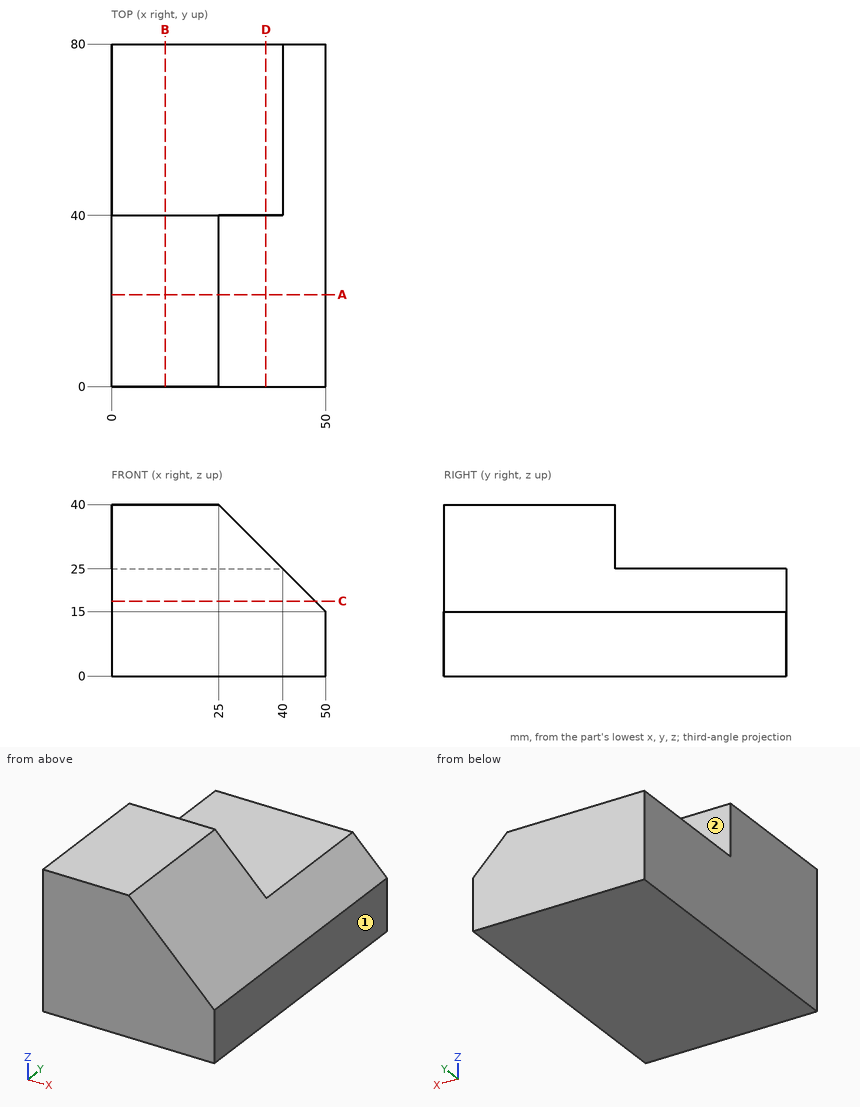
Design review of the part shown in the three views and the two pictorial views. Dimensions are in mm from the part's minimum x, y and z. A direction names the side the tool comes from. Give positions to 0.01 mm unless a question says otherwise; leave off trailing zeros. Write each loop counter-clockwise with the first axis right and the second up, starting at its lowest first coordinate (ties: lowest second). Pieces come first, ordered by that corner, then holes. Notation, with made-up numbers: M -31.75,-8.75 L 9.25,-8.75 A17 cw 9.25,4.25 Z; hole C -21,23 d3. An arc over 180 degrees is marked long. One line per question, with ' | ' between items. Start each with the question number.
Item 1: For the marked faces 1 and 2, list the 3-axis set-ups (+Z, -Z, +X, -X, +Y, -Y) from which the entire face can be reached by the end or side of a thin tool; tool diameter is ignored.
Item 2: For pin 1 (2 mm diameter, centred on y = 58.5, z = 24.5, fed in from +X); pin 2 (2 mm diameter, centred on x = 25, y = 47.5, fed in from +Z), all flat-tipped, find the tip position at first contact; note any pin that passes through.
Item 3: We need section A-A on y = 21.5. Write out the cut boundary in (x, z).
Item 4: We need section D-D on x = 36. Write out the cut boundary in (y, z).
Item 5: We need section C-C on z = 17.5. Write out the cut boundary in (x, y), plus the area to 3 significant figures.
Item 6: Wall thickness on line 1 (Z direction, x = 9, y = 48); line 2 (Y direction, x = 13, z = 29.5); line 3 (X direction, y = 20, z = 37): over which ranges is each line inside the solid? List them lowest first. Write a range as from..to.
Item 7: We need section B-B on x = 12.5. Write out the cut boundary in (y, z), plus the area to 3 significant figures.
Results found:
1) face 1: +Z, -Z, +X, +Y, -Y | face 2: +Z, +X, -X, +Y
2) pin 1: stops at x = 41.5 | pin 2: stops at z = 25
3) outline: M 0,0 L 50,0 L 50,15 L 25,40 L 0,40 Z
4) outline: M 0,0 L 80,0 L 80,25 L 40,25 L 40,29 L 0,29 Z
5) outline: M 0,0 L 47.5,0 L 47.5,80 L 0,80 Z | area: 3,800 mm2
6) line 1: z = 0..25 | line 2: y = 0..40 | line 3: x = 0..28
7) outline: M 0,0 L 80,0 L 80,25 L 40,25 L 40,40 L 0,40 Z | area: 2,600 mm2
